Here's how the part is built. I have some questions about the finished solid (model axes, mm). A direction names the side the tool comes from. Coordinates: 2 decimals unless noted, no trailing zeros. Write each loop counter-clockwise with the first axis right and the second up, starting at its lowest first coordinate (ties: lowest second). Pieces come first, ordered by that corner, then holes. Notation, with made-up numbers: (78.25, 73) -> (127.25, 73) arc R19 ccw to (127.25, 109) -> close; hole circle Ø2 at (53.25, 78.25). An arc over 180 degrees is marked (long way). Use a Markdown table: item, result. Add a question column.
Item 1: If we mould it in two halves opening along X, with no side actions, what happens to faces 1 (the flat face through (20, 25, -2)), 2 (the flat face through (0, 33, -2)), 3 (the flat face through (0, 34, -5))? For each: pulls with the +X half, pulls with the -X half, needs draft (parallel to the pull), parting line crosses it, or undercut.
Item 2: Imagine slicing it at D-D, the plane z = -0.45. Write out the boundary of the cut face in (x, y).
Item 3: Imagine slicing it at C-C, the plane y = 9. Write out the boundary of the cut face in (x, z), and give its area (3 significant figures).
Item 4: If I drill on line 1 along X through (y, z) = (17, -4.1); line 2 along Z through (x, y) = (17.6, 19); line 3 along Y through (x, z) = (-15.5, -3.65), over which ranges is the centre line in solid material (lowest first)? Write a range as from..to.
Item 5: On a 3-axis mill with a long thin cutter (end or side, diameter ignored), from which of +Z, -Z, +X, -X, +Y, -Y can I reach the whole of each face in a straight line? I mean faces 4 (the cylindrical face through (18.285, 19.217, -3.476)), 5 (the cylindrical face through (-18.285, 9.217, -3.476)), 6 (the flat face through (-15, 7, -2)), 7 (the cylindrical face through (-10, 31, -3)), 8 (the cylindrical face through (-14, 9, -2)). Say none if no direction works.
Item 6: Imagine slicing it at B-B, the plane x = 15.5. Write out the boundary of the cut face in (y, z).
Item 7: Imagine slicing it at A-A, the plane y = 32. Write out the boundary of the cut face in (x, z).
Item 8: Will these pins go through, and if not, where does the flat tip stop? pin 1 Ø2.5 at (x, y) = (-15.5, 19) entering from -Z; pin 2 Ø1.5 at (x, z) = (-1.5, -1) entering from -Y; pin 3 Ø1.8 at (y, z) = (9, -2.5) entering from -X.
```python
from build123d import *

# Parameters (mm, degrees)
F0_R     = 1.5
F1_DEPTH = 5
F3_D     = 2
F3_DEPTH = 5
F3_TIP   = 0.600860619
F4_R     = 5
F5_D     = 3


# Not quite as in the source:
# - a feature names something its author has since deleted; it is built from what else it names


with BuildPart() as f1:
    # F0 (on Top) → F1 (new body)
    with BuildSketch(Plane.XY):
        Polygon((11, 33), (11, 7), (20, 7), (20, 44), (0, 44), (0, 33), align=None)
        with Locations((15.5, 9)):
            Circle(F0_R, mode=Mode.SUBTRACT)
        with Locations((15.5, 19)):
            Circle(F0_R, mode=Mode.SUBTRACT)
    extrude(amount=-F1_DEPTH)

    # F3
    with Locations(Plane.YZ.offset(20)):
        with Locations((9, -2.5), (19, -2.5)):
            Hole(F3_D / 2, depth=F3_DEPTH)
            with Locations((0, 0, -(F3_DEPTH + F3_TIP / 2))):  # 118° drill point
                Cone(0, F3_D / 2, F3_TIP, mode=Mode.SUBTRACT)

    # F4
    f4_edges = [f1.edges().sort_by_distance(p)[0] for p in [
        (11, 33, -2.5),
    ]]
    fillet(f4_edges, radius=F4_R)

    # F5 (through all)
    with Locations(Plane.YZ.offset(20)):
        with Locations((14, -2.5)):
            Hole(F5_D / 2)

    # F6: F1 across plane


with BuildPart() as f1_1:
    add(f1.part)
    add(f1.part.mirror(Plane.YZ))


solid = f1_1.part
```
Ans:
| question | item | result |
|---|---|---|
| 1 | face 1 | pulls with the +X half |
| 1 | face 2 | undercut |
| 1 | face 3 | needs draft |
| 2 | outline | (-20, 7) -> (-11, 7) -> (-11, 28) arc R5 cw to (-6, 33) -> (6, 33) arc R5 cw to (11, 28) -> (11, 7) -> (20, 7) -> (20, 44) -> (-20, 44) -> close; hole circle Ø3 at (-15.5, 9); hole circle Ø3 at (-15.5, 19); hole circle Ø3 at (15.5, 9); hole circle Ø3 at (15.5, 19) |
| 3 | outline | (-20, -5) -> (-17, -5) -> (-17, -3.5) -> (-20, -3.5) -> close; (-20, -1.5) -> (-17, -1.5) -> (-17, 0) -> (-20, 0) -> close; (-14, -5) -> (-11, -5) -> (-11, 0) -> (-14, 0) -> close; (11, -5) -> (14, -5) -> (14, 0) -> (11, 0) -> close; (17, -5) -> (20, -5) -> (20, -3.5) -> (17, -3.5) -> close; (17, -1.5) -> (20, -1.5) -> (20, 0) -> (17, 0) -> close |
| 3 | area | 48.0 mm^2 |
| 4 | line 1 | x = -20..-11, 11..20 |
| 4 | line 2 | z = -5..-3.5, -1.5..0 |
| 4 | line 3 | y = 7..7.5, 10.5..13.04, 14.96..17.5, 20.5..44 |
| 5 | face 4 | +X |
| 5 | face 5 | -X |
| 5 | face 6 | +Z, -Z, +X, -X, -Y |
| 5 | face 7 | +Z, -Z, -Y |
| 5 | face 8 | +Z, -Z |
| 6 | outline | (7, -5) -> (7.5, -5) -> (7.5, 0) -> (7, 0) -> close; (10.5, -5) -> (17.5, -5) -> (17.5, 0) -> (10.5, 0) -> close; (20.5, -5) -> (44, -5) -> (44, 0) -> (20.5, 0) -> close; hole circle Ø3 at (14, -2.5) |
| 7 | outline | (-20, -5) -> (-9, -5) -> (-9, 0) -> (-20, 0) -> close; (9, -5) -> (20, -5) -> (20, 0) -> (9, 0) -> close |
| 8 | pin 1 | passes through |
| 8 | pin 2 | stops at y = 33 |
| 8 | pin 3 | stops at x = -14.3 |
